Here's how the part is built. I have some questions about the finished solid (model axes, mm). Coordinates: 2 decimals unless noted, no trailing zeros. Write each loop counter-clockwise with the first axis right and the second up, starting at its lowest first coordinate (ties: lowest second). Pieces come first, ordered by that corner, then holes.
(1) Please list where these lines run through material, in increasing order: probe 1 along X at (y, z) = (177.5, 8.85); probe 2 along Y at (x, z) = (6.5, 8.4); probe 3 along Y at (x, z) = (98.5, 2.9).
(2) For pin 1 Ø8 at (x, y) = (38.5, 147.5) entering from -Z; pin 2 Ø7 at (x, y) = (85.5, 22.5) entering from +Z, each with a flat end and sliding along its axis, tell me the tip position at first contact or that it passes through.
(3) Imagine slicing it at A-A, the plane x = 22. List the corners of the cut face in (y, z) for me, plus the area to 3 significant figures.
(4) Imagine slicing it at B-B, the plane y = 23. List the corners of the cut face in (x, z) for me.
(5) Imagine slicing it at C-C, the plane x = 6.5. State how many separate pieces and enclosed holes the cut face has, plus the area to 3 significant figures.
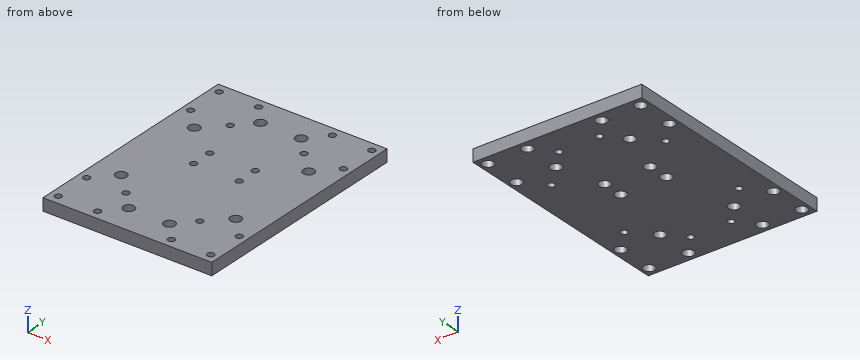
```python
from build123d import *

# Parameters (mm, degrees)
SZKIC1_W                                             = 137
SZKIC1_H                                             = 185
DODANIE_WYCI_GNI_CIE1_DEPTH                          = 10
POG_BIENIE_WALCOWE_POD_M5_WKR_T_DO_CZ_CI_D           = 5.5
POG_BIENIE_WALCOWE_POD_M5_WKR_T_DO_CZ_CI_CBORE_D     = 9
POG_BIENIE_WALCOWE_POD_M5_WKR_T_DO_CZ_CI_CBORE_DEPTH = 6
POG_BIENIE_WALCOWE_POD_M5_WKR_T_DO_C_2_D             = 5.5
POG_BIENIE_WALCOWE_POD_M5_WKR_T_DO_C_2_CBORE_D       = 9
POG_BIENIE_WALCOWE_POD_M5_WKR_T_DO_C_2_CBORE_DEPTH   = 6
POG_BIENIE_WALCOWE_POD_M5_WKR_T_DO_C_3_D             = 5.5
POG_BIENIE_WALCOWE_POD_M5_WKR_T_DO_C_3_CBORE_D       = 9
POG_BIENIE_WALCOWE_POD_M5_WKR_T_DO_C_3_CBORE_DEPTH   = 6


with BuildPart() as part:
    # Szkic1 → Dodanie-wyciągnięcie1 (new body)
    with BuildSketch(Plane.XY):
        with Locations((68.5, 92.5)):
            Rectangle(SZKIC1_W, SZKIC1_H)
    extrude(amount=DODANIE_WYCI_GNI_CIE1_DEPTH)

    # Pog_bienie walcowe pod M5 Wkr_t do cz_ci (through all)
    with Locations(Plane(origin=(0, 0, 0), x_dir=(-1, 0, 0), z_dir=(0, 0, -1))):
        with Locations((-38.5, 177.5), (-6.5, 177.5), (-38.5, 147.5), (-6.5, 147.5), (-38.5, 37.5), (-6.5, 37.5), (-38.5, 7.5), (-6.5, 7.5), (-130.5, 7.5), (-98.5, 7.5), (-130.5, 37.5), (-98.5, 37.5), (-130.5, 147.5), (-98.5, 147.5), (-130.5, 177.5), (-98.5, 177.5)):
            CounterBoreHole(POG_BIENIE_WALCOWE_POD_M5_WKR_T_DO_CZ_CI_D / 2, POG_BIENIE_WALCOWE_POD_M5_WKR_T_DO_CZ_CI_CBORE_D / 2, POG_BIENIE_WALCOWE_POD_M5_WKR_T_DO_CZ_CI_CBORE_DEPTH)

    # Pog_bienie walcowe pod M5 Wkr_t do c 2 (through all)
    with Locations(Plane.XY.offset(10)):
        with Locations((52, 162), (22, 131), (22, 54), (52, 23), (85, 23), (115, 54), (115, 131), (85, 162)):
            CounterBoreHole(POG_BIENIE_WALCOWE_POD_M5_WKR_T_DO_C_2_D / 2, POG_BIENIE_WALCOWE_POD_M5_WKR_T_DO_C_2_CBORE_D / 2, POG_BIENIE_WALCOWE_POD_M5_WKR_T_DO_C_2_CBORE_DEPTH)

    # Pog_bienie walcowe pod M5 Wkr_t do c 3 (through all)
    with Locations(Plane(origin=(0, 0, 0), x_dir=(-1, 0, 0), z_dir=(0, 0, -1))):
        with Locations((-87, 111), (-50, 111), (-87, 94), (-50, 94)):
            CounterBoreHole(POG_BIENIE_WALCOWE_POD_M5_WKR_T_DO_C_3_D / 2, POG_BIENIE_WALCOWE_POD_M5_WKR_T_DO_C_3_CBORE_D / 2, POG_BIENIE_WALCOWE_POD_M5_WKR_T_DO_C_3_CBORE_DEPTH)


solid = part.part
```
Recorded:
1. probe 1: x = 0 to 3.75, 9.25 to 35.75, 41.25 to 95.75, 101.25 to 127.75, 133.25 to 137
1. probe 2: y = 0 to 4.75, 10.25 to 34.75, 40.25 to 144.75, 150.25 to 174.75, 180.25 to 185
1. probe 3: y = 0 to 3, 12 to 33, 42 to 143, 152 to 173, 182 to 185
2. pin 1: stops at z = 6
2. pin 2: stops at z = 4
3. outline: (0, 0) - (51.25, 0) - (51.25, 4) - (49.5, 4) - (49.5, 10) - (0, 10) - close; (56.75, 0) - (128.25, 0) - (128.25, 4) - (126.5, 4) - (126.5, 10) - (58.5, 10) - (58.5, 4) - (56.75, 4) - close; (133.75, 0) - (185, 0) - (185, 10) - (135.5, 10) - (135.5, 4) - (133.75, 4) - close
3. area: 1,700 mm2
4. outline: (0, 0) - (49.25, 0) - (49.25, 4) - (47.5, 4) - (47.5, 10) - (0, 10) - close; (54.75, 0) - (82.25, 0) - (82.25, 4) - (80.5, 4) - (80.5, 10) - (56.5, 10) - (56.5, 4) - (54.75, 4) - close; (87.75, 0) - (137, 0) - (137, 10) - (89.5, 10) - (89.5, 4) - (87.75, 4) - close
5. separate pieces: 5
5. enclosed holes: 0
5. area: 1,550 mm2
